```python
from build123d import *

# Parameters (mm, degrees)
WALLS_DEPTH               = 1.6
WALLS_DEPTH_BACK          = 18
PORTS_REACH               = 81.148
PORT_SKETCH_W             = 14
PORT_SKETCH_H             = 4.5
PORT_SKETCH_W_2           = 13
PORT_FILLET_R             = 0.5
MOUNTING_BASE_START       = -11.07
MOUNTING_BASE_SKETCH_R    = 2.5
MOUNTING_BASE_DEPTH       = 12.67
MOUNTING_PINS_START       = -18
MOUNTING_BASE_SKETCH_2_R  = 2.5
MOUNTING_PINS_DEPTH       = 19.6
MOUNTING_PIN_CHAMFER_SIZE = 0.5


with BuildPart() as part:
    # Base_Sketch → Walls (new, two sides: drawn at the far end of the back side and taken through both)
    with BuildSketch(Plane(origin=(0, -11.07, 0), x_dir=(-1, 0, 0), z_dir=(0, -1, 0)).offset(-WALLS_DEPTH_BACK)):
        with BuildLine():
            Line((-32.98, 16.51), (-32.98, -36.83))
            ThreePointArc((-32.98, -36.83), (-31.503818177, -40.393818177), (-27.94, -41.87))
            Line((-27.94, -41.87), (27.94, -41.87))
            ThreePointArc((27.94, -41.87), (31.503818177, -40.393818177), (32.98, -36.83))
            Line((32.98, -36.83), (32.98, 36.83))
            ThreePointArc((32.98, 36.83), (31.503818177, 40.393818177), (27.94, 41.87))
            Line((27.94, 41.87), (-7.62, 41.87))
            ThreePointArc((-7.62, 41.87), (-9.548724499, 41.486352844), (-11.183818177, 40.393818177))
            Line((-11.183818177, 40.393818177), (-31.503818177, 20.073818177))
            ThreePointArc((-31.503818177, 20.073818177), (-32.596352844, 18.438724499), (-32.98, 16.51))
        make_face()
        with BuildLine():
            Line((-30.98, 16.51), (-30.98, -36.83))
            ThreePointArc((-30.98, -36.83), (-30.089604615, -38.979604615), (-27.94, -39.87))
            Line((-27.94, -39.87), (27.94, -39.87))
            ThreePointArc((27.94, -39.87), (30.089604615, -38.979604615), (30.98, -36.83))
            Line((30.98, -36.83), (30.98, 36.83))
            ThreePointArc((30.98, 36.83), (30.089604615, 38.979604615), (27.94, 39.87))
            Line((27.94, 39.87), (-7.62, 39.87))
            ThreePointArc((-7.62, 39.87), (-8.783357634, 39.638593779), (-9.769604615, 38.979604615))
            Line((-9.769604615, 38.979604615), (-30.089604615, 18.659604615))
            ThreePointArc((-30.089604615, 18.659604615), (-30.748593779, 17.673357634), (-30.98, 16.51))
        make_face(mode=Mode.SUBTRACT)
    extrude(amount=WALLS_DEPTH + WALLS_DEPTH_BACK)

    # Port_Sketch → Ports (cut, up to next)
    with BuildSketch(Plane.ZY.offset(32.98), mode=Mode.PRIVATE) as ports_sk1:
        with Locations((7.61, 4.68)):
            Rectangle(PORT_SKETCH_W, PORT_SKETCH_H)
    ports_tool1 = extrude(ports_sk1.sketch, amount=-PORTS_REACH, mode=Mode.PRIVATE) & part.part
    # Port_Sketch → Ports (cut, up to next)
    with BuildSketch(Plane.ZY.offset(32.98), mode=Mode.PRIVATE) as ports_sk2:
        with Locations((-24.97, 4.68)):
            Rectangle(PORT_SKETCH_W_2, PORT_SKETCH_H)
    ports_tool2 = extrude(ports_sk2.sketch, amount=-PORTS_REACH, mode=Mode.PRIVATE) & part.part
    add(ports_tool1.solids().sort_by_distance((-32.98, 4.68, 7.61))[0], mode=Mode.SUBTRACT)
    add(ports_tool2.solids().sort_by_distance((-32.98, 4.68, -24.97))[0], mode=Mode.SUBTRACT)

    # Port_Fillet
    port_fillet_edges = [part.edges().sort_by_distance(p)[0] for p in [
        (-31.98, 6.93, -18.47),
        (-31.98, 6.93, -31.47),
        (-31.98, 2.43, -31.47),
        (-31.98, 2.43, -18.47),
        (-31.98, 2.43, 0.61),
        (-31.98, 6.93, 0.61),
        (-31.98, 6.93, 14.61),
        (-31.98, 2.43, 14.61),
    ]]
    fillet(port_fillet_edges, radius=PORT_FILLET_R)

    # Mounting_Base_Sketch → Mounting_Base (add)
    # profile 1 of 3: a face of its own
    with BuildSketch(Plane(origin=(0, -11.07, 0), x_dir=(-1, 0, 0), z_dir=(0, -1, 0)).offset(MOUNTING_BASE_START)):
        with BuildLine():
            Line((22.400144884, -34.290144884), (22.400144884, -39.87))
            Line((22.400144884, -39.87), (25.400144884, -39.87))
            Line((25.400144884, -39.87), (25.400144884, -37.290144884))
            ThreePointArc((25.400144884, -37.290144884), (27.521465228, -36.411465228), (28.400144884, -34.290144884))
            Line((28.400144884, -34.290144884), (30.98, -34.290144884))
            Line((30.98, -34.290144884), (30.98, -31.290144884))
            Line((30.98, -31.290144884), (25.400144884, -31.290144884))
            ThreePointArc((25.400144884, -31.290144884), (23.27882454, -32.16882454), (22.400144884, -34.290144884))
        make_face()
        with Locations(Location((25.400144884, -34.290144884, 0), (0, 0, 270))):
            Circle(MOUNTING_BASE_SKETCH_R, mode=Mode.SUBTRACT)
    # profile 2 of 3: a face of its own
    with BuildSketch(Plane(origin=(0, -11.07, 0), x_dir=(-1, 0, 0), z_dir=(0, -1, 0)).offset(MOUNTING_BASE_START)):
        with BuildLine():
            Line((-25.400144884, -31.290144884), (-30.98, -31.290144884))
            Line((-30.98, -31.290144884), (-30.98, -34.290144884))
            Line((-30.98, -34.290144884), (-28.400144884, -34.290144884))
            ThreePointArc((-28.400144884, -34.290144884), (-27.521465228, -36.411465228), (-25.400144884, -37.290144884))
            Line((-25.400144884, -37.290144884), (-25.400144884, -39.87))
            Line((-25.400144884, -39.87), (-22.400144884, -39.87))
            Line((-22.400144884, -39.87), (-22.400144884, -34.290144884))
            ThreePointArc((-22.400144884, -34.290144884), (-23.27882454, -32.16882454), (-25.400144884, -31.290144884))
        make_face()
        with Locations(Location((-25.400144884, -34.290144884, 0), (0, 0, 270))):
            Circle(MOUNTING_BASE_SKETCH_R, mode=Mode.SUBTRACT)
    # profile 3 of 3: a face of its own
    with BuildSketch(Plane(origin=(0, -11.07, 0), x_dir=(-1, 0, 0), z_dir=(0, -1, 0)).offset(MOUNTING_BASE_START)):
        with BuildLine():
            Line((22.400144884, 34.290144884), (22.400144884, 39.87))
            Line((22.400144884, 39.87), (25.400144884, 39.87))
            Line((25.400144884, 39.87), (25.400144884, 37.290144884))
            ThreePointArc((25.400144884, 37.290144884), (27.521465228, 36.411465228), (28.400144884, 34.290144884))
            Line((28.400144884, 34.290144884), (30.98, 34.290144884))
            Line((30.98, 34.290144884), (30.98, 31.290144884))
            Line((30.98, 31.290144884), (25.400144884, 31.290144884))
            ThreePointArc((25.400144884, 31.290144884), (23.27882454, 32.16882454), (22.400144884, 34.290144884))
        make_face()
        with Locations(Location((25.400144884, 34.290144884, 0), (0, 0, 270))):
            Circle(MOUNTING_BASE_SKETCH_R, mode=Mode.SUBTRACT)
    extrude(amount=MOUNTING_BASE_DEPTH)

    # Mounting_Base_Sketch<2> → Mounting_Pins (add)
    with BuildSketch(Plane(origin=(0, -11.07, 0), x_dir=(-1, 0, 0), z_dir=(0, -1, 0)).offset(MOUNTING_PINS_START)):
        with Locations(Location((-25.400144884, -34.290144884, 0), (0, 0, 90))):
            Circle(MOUNTING_BASE_SKETCH_2_R)
        with Locations(Location((25.400144884, -34.290144884, 0), (0, 0, 90))):
            Circle(MOUNTING_BASE_SKETCH_2_R)
        with Locations(Location((25.400144884, 34.290144884, 0), (0, 0, 90))):
            Circle(MOUNTING_BASE_SKETCH_2_R)
    extrude(amount=MOUNTING_PINS_DEPTH)

    # Mounting_Pin_Chamfer
    mounting_pin_chamfer_edges = [part.edges().sort_by_distance(p)[0] for p in [
        (25.400144884, 0, 36.790144884),
        (-25.400144884, 0, 36.790144884),
        (-25.400144884, 0, -31.790144884),
        (25.400144884, 6.93, 36.790144884),
        (-25.400144884, 6.93, 36.790144884),
        (-25.400144884, 6.93, -31.790144884),
    ]]
    chamfer(mounting_pin_chamfer_edges, length=MOUNTING_PIN_CHAMFER_SIZE - 0.0001)  # a hair under: the kernel refuses the full size


solid = part.part
```
Input: part model. Units: mm. Frame: model coordinates. A direction names the side the tool comes from. Give positions to 0.01 mm unless a question says otherwise; leave off trailing zeros. Write each loop counter-clockwise with the first axis right and the second up, starting at its lowest first coordinate (ties: lowest second). Pieces come first, ordered by that corner, then holes. Notation, with made-up numbers: (-24.5, 9.25) - (-3.5, 9.25) arc R25 cw to (-3.5, 24.25) - close; hole circle Ø8 at (-22, 7.25). An arc over 180 degrees is marked (long way). Write item = value, one per line. Start each with the question number.
1. Section query A-A, the plane z = 21. Output: boundary loops of the cut face in (x, y), then the cut area to 3 significant figures.
2. Ray query, L1, parallel to X at y = 1.25, z = 18.5; L2, parallel to Z at x = 26, y = 0.25; L3, parallel to Z at x = -13, y = -7.5. Return the intervals inside material, ascending.
3. Mould query, pull axis Z, two halves, no side actions, for faces 1 (the cylindrical face through (31.5, -2.7, 40.4)), 2 (the flat face through (-30, -6, 34.29)), 3 (the flat face through (21.2, -2.73, -30.38)). Classes: released by +Z, released by -Z, zero draft, split by the parting line, or undercut.
4. Section query B-B, the plane x = -4.5. Output: boundary loops of the cut face in (y, z), then the cut area to 3 significant figures.
5. Section query C-C, the plane y = -4.5. Count the separate pieces of the cut face and the enclosed holes in it, then the cut area to 3 significant figures.
6. First-contact query: pin 1 Ø2 at (x, y) = (-31.5, 5) entering from +Z; pin 2 Ø3 at (x, y) = (28.5, -8) entering from -Z; pin 3 Ø1 at (x, z) = (-32.5, -25.5) entering from +Y. Flat tips, straight axial feed; report the tip coordinate or a pass-through.
7. Access query for faces 4 (the flat face through (-32, 5, 0.61)), 5 (the flat face through (-25, 6.93, 34)), 6 (the flat face through (30, -6, 34.29)). Directions: +Z, -Z, +X, -X, +Y, -Y. A direction counts if a zero-diameter tool reaches every point of the face in a straight line with its end or side. Return the directions, or none.
Check sheet entries:
q1.outline = (-32.98, -12.67) - (-30.98, -12.67) - (-30.98, 6.93) - (-32.98, 6.93) - close; (30.98, -12.67) - (32.98, -12.67) - (32.98, 6.93) - (30.98, 6.93) - close
q1.area = 78.4 mm2
q2.L1 = -32.98 to -30.98, 30.98 to 32.98
q2.L2 = -25.58 to -22.75, 31.61 to 36.97, 39.87 to 41.87
q2.L3 = -41.87 to -39.87, 39.87 to 41.87
q3.face_1 = released by +Z
q3.face_2 = undercut
q3.face_3 = released by -Z
q4.outline = (-12.67, -41.87) - (6.93, -41.87) - (6.93, -39.87) - (-12.67, -39.87) - close; (-12.67, 39.87) - (6.93, 39.87) - (6.93, 41.87) - (-12.67, 41.87) - close
q4.area = 78.4 mm2
q5.separate_pieces = 1
q5.enclosed_holes = 4
q5.area = 688 mm2
q6.pin_1 = 41.17
q6.pin_2 = -24.58
q6.pin_3 = 2.43
q7.face_4 = -X, +Y
q7.face_5 = +Z, -Z, +X, -X, +Y
q7.face_6 = +Y, -Y
